Design review of the part built by this model. Coordinates are the model's own, in mm. A direction names the side the tool comes from. Give positions to 0.01 mm unless a question says otherwise; leave off trailing zeros. Loops run counter-clockwise (first coordinate to the right, second up) from the corner with the lowest first, then second, coordinate; pieces in that order, holes last.
from build123d import *

# Parameters (mm, degrees)
SKETCH_1_W          = 100
SKETCH_1_H          = 68
EXTRUDE_1_DEPTH     = 2
SKETCH_2_R          = 1
CUT_EXTRUDE_1_DEPTH = 2
SKETCH_3_R          = 2
CUT_EXTRUDE_2_DEPTH = 1.5
SKETCH_4_W          = 74
SKETCH_4_H          = 49.6
CUT_EXTRUDE_3_DEPTH = 5
FILLET_1_R          = 1
FILLET_2_R          = 1
FILLET_3_R          = 0.2


with BuildPart() as part:
    # Эскиз1 → Бобышка-Вытянуть1 (new body)
    with BuildSketch(Plane(origin=(0, 0, 0), x_dir=(1, 0, 0), z_dir=(0, 1, 0))):
        Rectangle(SKETCH_1_W, SKETCH_1_H)
    extrude(amount=EXTRUDE_1_DEPTH)

    # Эскиз2 → Вырез-Вытянуть1 (cut)
    with BuildSketch(Plane(origin=(0, 2, 0), x_dir=(1, 0, 0), z_dir=(0, 1, 0))):
        with Locations(Location((-46, 31.5, 0), (0, 0, 270))):
            Circle(SKETCH_2_R)
        with Locations(Location((33, 31.5, 0), (0, 0, 90))):
            Circle(SKETCH_2_R)
        with Locations(Location((33, -31.5, 0), (0, 0, 270))):
            Circle(SKETCH_2_R)
        with Locations(Location((-46, -31.5, 0), (0, 0, 90))):
            Circle(SKETCH_2_R)
    extrude(amount=-CUT_EXTRUDE_1_DEPTH, mode=Mode.SUBTRACT)

    # Эскиз3 → Вырез-Вытянуть2 (cut)
    with BuildSketch(Plane(origin=(0, 2, 0), x_dir=(1, 0, 0), z_dir=(0, 1, 0))):
        with Locations(Location((-46, 31.5, 0), (0, 0, 270))):
            Circle(SKETCH_3_R)
        with Locations(Location((-46, -31.5, 0), (0, 0, 270))):
            Circle(SKETCH_3_R)
        with Locations(Location((33, -31.5, 0), (0, 0, 270))):
            Circle(SKETCH_3_R)
        with Locations(Location((33, 31.5, 0), (0, 0, 270))):
            Circle(SKETCH_3_R)
    extrude(amount=-CUT_EXTRUDE_2_DEPTH, mode=Mode.SUBTRACT)

    # Эскиз4 → Вырез-Вытянуть3 (cut)
    with BuildSketch(Plane(origin=(0, 2, 0), x_dir=(1, 0, 0), z_dir=(0, 1, 0))):
        with Locations((-7.5, 0)):
            Rectangle(SKETCH_4_W, SKETCH_4_H)
    extrude(amount=-CUT_EXTRUDE_3_DEPTH, mode=Mode.SUBTRACT)

    # Скругление1
    fillet_1_edges = [part.edges().sort_by_distance(p)[0] for p in [
        (-7.5, 2, -24.8),
        (-50, 2, 0),
        (-50, 0, 0),
    ]]
    fillet(fillet_1_edges, radius=FILLET_1_R - 0.0001)  # a hair under: the kernel refuses the full size

    # Скругление2
    fillet_2_edges = [part.edges().sort_by_distance(p)[0] for p in [
        (-44.5, 2, -0.49995),
        (-7.5, 2, 24.8),
        (29.5, 2, -0.49995),
    ]]
    fillet(fillet_2_edges, radius=FILLET_2_R - 0.0001)  # a hair under: the kernel refuses the full size

    # Скругление3
    fillet_3_edges = [part.edges().sort_by_distance(p)[0] for p in [
        (-46, 2, -33.5),
        (-46, 2, 29.5),
        (33, 2, 29.5),
        (33, 2, -33.5),
    ]]
    fillet(fillet_3_edges, radius=FILLET_3_R)


solid = part.part
Q1. Insertion check: pin 1 (1.8 mm diameter, centred on x = -46, z = -31.5, fed in from -Y); pin 2 (6.5 mm diameter, centred on x = 33, z = -31.5, fed in from -Y); pin 3 (3 mm diameter, centred on x = -46, z = -31.5, fed in from +Y). Each pin has a flat end and moves straight along its axis. Give the tip position at first contact, or say it passes through.
Results:
pin 1: passes through
pin 2: stops at y = 0
pin 3: stops at y = 0.5
Q2. Take a section at C-C (x = 33). Give the boundary of the cut face in (y, z), plus the area to 3 significant figures.
Results:
outline: (0, -34) - (2, -34) - (2, -33.7) arc R0.2 ccw to (1.8, -33.5) - (0.5, -33.5) - (0.5, -32.5) - (0, -32.5) - close; (0, -30.5) - (0.5, -30.5) - (0.5, -29.5) - (1.8, -29.5) arc R0.2 ccw to (2, -29.3) - (2, 29.3) arc R0.2 ccw to (1.8, 29.5) - (0.5, 29.5) - (0.5, 30.5) - (0, 30.5) - close; (0, 32.5) - (0.5, 32.5) - (0.5, 33.5) - (1.8, 33.5) arc R0.2 ccw to (2, 33.7) - (2, 34) - (0, 34) - close
area: 122 mm2
Q3. Take a section at B-B (z = -31.5). Give the number of separate pieces and of enclosed holes in the cut face, plus the area to 3 significant figures.
Results:
separate pieces: 3
enclosed holes: 0
area: 186 mm2
Q4. Tool access review of faces 1 (the face through (31.226, 1.159, 32.423)), 2 (the face through (32.01, 0.25, -31.37)): name each direction out of +Z, -Z, +X, -X, +Y, -Y from which nothing blocks a thin tool from reaching the whole face with its end or side.
Results:
face 1: +Y
face 2: +Y, -Y
Q5. Wall thickness on line 1 (X direction, y = 1.2, z = 31.5); line 2 (Z direction, x = -36, y = 0.5); line 3 (X direction, y = 1, z = -12): over which ranges is each line inside the solid? List them lowest first.
Results:
line 1: x = -49.98 to -48, -44 to 31, 35 to 50
line 2: z = -34 to -24.8, 24.8 to 34
line 3: x = -50 to -44.5, 29.5 to 50
Q6. Draft analysis for pull direction X (two halves, no side actions). For faces 3 (the face through (50, 1, 0)), 4 (the face through (32.1, 0.5, 32.4)), 5 (the face through (33, 2, 2)), state which applies: pulls with the +X half, pulls with the -X half, needs draft (parallel to the pull), parting line crosses it, or undercut.
Results:
face 3: pulls with the +X half
face 4: undercut
face 5: needs draft
Q7. Take a section at A-A (x = 2.5). Give the boundary of the cut face in (y, z).
Results:
outline: (0, -34) - (2, -34) - (2, -25.8) arc R1 ccw to (1, -24.8) - (0, -24.8) - close; (0, 24.8) - (1, 24.8) arc R1 ccw to (2, 25.8) - (2, 34) - (0, 34) - close
